Design review of the part shown in the three views and the two pictorial views. Dimensions are in mm from the part's minimum x, y and z. A direction names the side the tool comes from. Coordinates: 2 decimals unless noted, no trailing zeros. Loops run counter-clockwise (first coordinate to the right, second up) from the corner with the lowest first, then second, coordinate; pieces in that order, holes last. Notation, with made-up numbers: (58.5, -2.5) -> (96.5, -2.5) arc R11 cw to (96.5, 6.5) -> close; hole circle Ø7 at (-37, -1). An arc over 180 degrees is marked (long way). One line per item, written item: value.
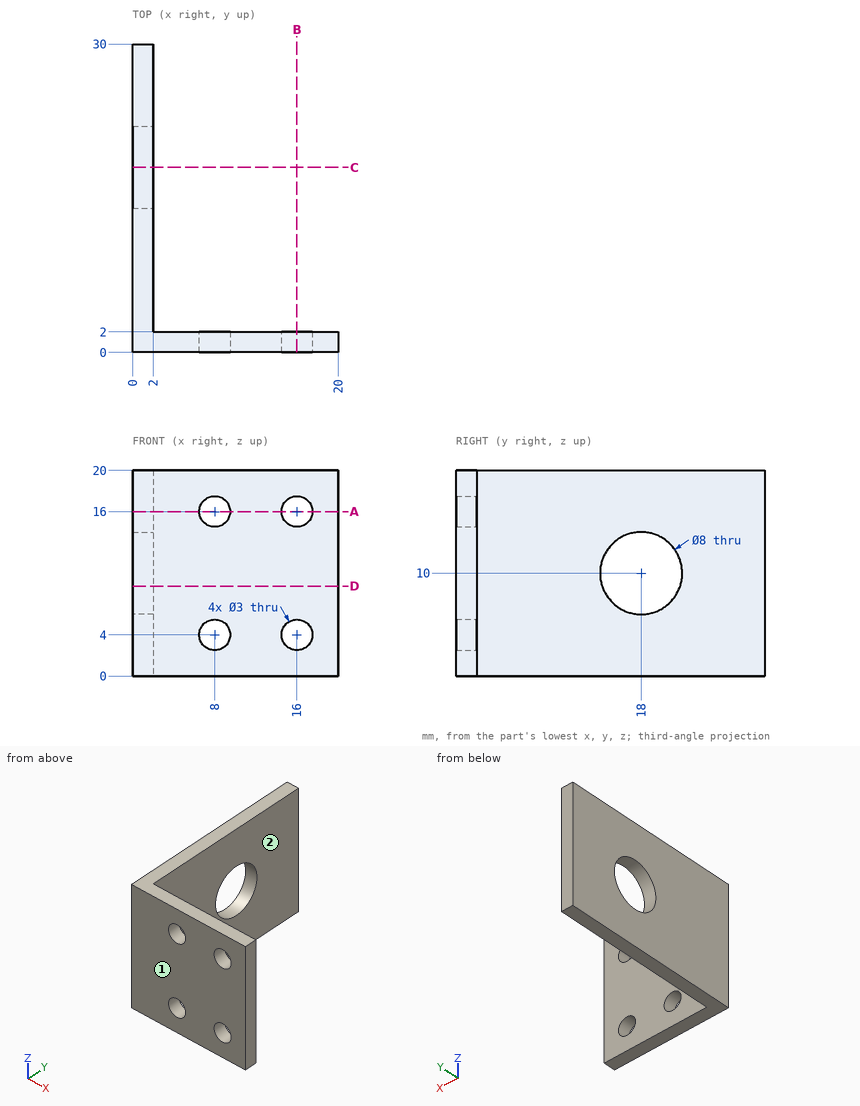
1. Take a section at B-B, the plane x = 16. Give the boundary of the cut face in (y, z).
Return value:
outline: (0, 0) -> (2, 0) -> (2, 2.5) -> (0, 2.5) -> close; (0, 5.5) -> (2, 5.5) -> (2, 14.5) -> (0, 14.5) -> close; (0, 17.5) -> (2, 17.5) -> (2, 20) -> (0, 20) -> close
2. Take a section at D-D, the plane z = 8.75. Give the boundary of the cut face in (x, y).
Return value:
outline: (0, 0) -> (20, 0) -> (20, 2) -> (2, 2) -> (2, 14.2) -> (0, 14.2) -> close; (0, 21.8) -> (2, 21.8) -> (2, 30) -> (0, 30) -> close
3. Take a section at C-C, the plane y = 18. Give the boundary of the cut face in (x, z).
Return value:
outline: (0, 0) -> (2, 0) -> (2, 6) -> (0, 6) -> close; (0, 14) -> (2, 14) -> (2, 20) -> (0, 20) -> close
4. To check wall thickness, follow probe 1 along Z at (x, y) = (8, 0.4); probe 2 along X at (y, z) = (0.75, 16); probe 3 along Y at (x, z) = (0.4, 10). State the ranges of each line that lie inside material, in increasing order. Write a range as from..to.
Return value:
probe 1: z = 0..2.5, 5.5..14.5, 17.5..20
probe 2: x = 0..6.5, 9.5..14.5, 17.5..20
probe 3: y = 0..14, 22..30
5. Take a section at A-A, the plane z = 16. Give the boundary of the cut face in (x, y).
Return value:
outline: (0, 0) -> (6.5, 0) -> (6.5, 2) -> (2, 2) -> (2, 30) -> (0, 30) -> close; (9.5, 0) -> (14.5, 0) -> (14.5, 2) -> (9.5, 2) -> close; (17.5, 0) -> (20, 0) -> (20, 2) -> (17.5, 2) -> close
6. For the marked faces 1 and 2, list the 3-axis set-ups (+Z, -Z, +X, -X, +Y, -Y) from which the entire face can be reached by the end or side of a thin tool; tool diameter is ignored.
Return value:
face 1: +Z, -Z, +X, -X, -Y
face 2: +Z, -Z, +X, +Y
7. Insertion check: pin 1 Ø5.5 at (x, z) = (10, 14.5) entering from +Y; pin 2 Ø1.8 at (x, z) = (8, 4) entering from +Y; pin 3 Ø6 at (y, z) = (9.5, 14.5) entering from +X. Each pin has a flat end and moves straight along its axis. Give the tip position at first contact, or say it passes through.
Return value:
pin 1: stops at y = 2
pin 2: passes through
pin 3: stops at x = 2
